```python
from build123d import *

# Parameters (mm, degrees)
CYLINDER003012_R     = 0.93
CYLINDER003012_DEPTH = 20
CYLINDER003013_R     = 2.4
CYLINDER003013_DEPTH = 4.5
CYLINDER003014_R     = 3.45
CYLINDER003014_DEPTH = 4.5


with BuildPart() as cylinder013:
    # Cylinder003012 → Cylinder003012 (new body)
    with BuildSketch(Plane(origin=(11, 10, -8), x_dir=(1, 0, 0), z_dir=(0, 0, 1))):
        Circle(CYLINDER003012_R)
    extrude(amount=CYLINDER003012_DEPTH)


with BuildPart() as cylinder014:
    # Cylinder003013 → Cylinder003013 (new body)
    with BuildSketch(Plane(origin=(11, 10, -0.5), x_dir=(1, 0, 0), z_dir=(0, 0, 1))):
        Circle(CYLINDER003013_R)
    extrude(amount=CYLINDER003013_DEPTH)


with BuildPart() as propeller_hub:
    # Cylinder003014 → Cylinder003014 (new body)
    with BuildSketch(Plane(origin=(11, 10, -4.5), x_dir=(1, 0, 0), z_dir=(0, 0, 1))):
        Circle(CYLINDER003014_R)
    extrude(amount=CYLINDER003014_DEPTH)

    # Fusion001: union Cylinder014
    add(cylinder014.part)

    # Cut002002002018: cut Cylinder013
    add(cylinder013.part, mode=Mode.SUBTRACT)


solid = propeller_hub.part
```
Verification items for the finished model (mm, model axes). A direction names the side the tool comes from. Coordinates: 2 decimals unless noted, no trailing zeros. Order: outer loops, then holes, each group sorted by start corner. A loop starts at its lowest first (then second) coordinate and runs counter-clockwise, first axis right, second up. Notation, with made-up numbers: (73.25, 34.5) -> (85.25, 34.5) arc R5 ccw to (85.25, 43.5) -> close; hole circle Ø7 at (-4.75, 63.25). An arc over 180 degrees is marked (long way). Put each result on its own line as item: value. Start each with the question number.
1) Tool access check on faces 4 (the flat face through (12, 9, -4.5)), 5 (the cylindrical face through (10.69, 12.38, 1.97)). Record the directions out of +Z, -Z, +X, -X, +Y, -Y that give a thin tool (end or side, any length) a straight path to the whole face; none if there is none.
2) Release check for a two-part mould opening along X. For faces 1 (the cylindrical face through (10.252, 6.632, -2.282)), 2 (the cylindrical face through (11.5, 10.784, -0.309)), 3 (the flat face through (12, 9.5, 4)) record: pulls with the +X half, pulls with the -X half, needs draft (parallel to the pull), parting line crosses it, or undercut.
3) Cross-section at D-D (y = 8). Enter the section's corners in (x, z).
4) Material ranges on L1, parallel to Y at x = 11, z = -1; L2, parallel to Z at x = 12.75, y = 12.5; L3, parallel to X at y = 10, z = 0.5, recorded low to high.
5) Cross-section at C-C (z = -2.5). Enter the section's corners in (x, y), plus the area to 3 significant figures.
6) Cross-section at B-B (y = 10). Enter the section's corners in (x, z).
7) Cross-section at A-A (x = 11). Enter the section's corners in (y, z).
Geometry check:
1. face 4: -Z, +X, -X, +Y, -Y
1. face 5: +Z
2. face 1: parting line crosses it
2. face 2: undercut
2. face 3: needs draft
3. outline: (8.19, -4.5) -> (13.81, -4.5) -> (13.81, 0) -> (12.33, 0) -> (12.33, 4) -> (9.67, 4) -> (9.67, 0) -> (8.19, 0) -> close
4. L1: y = 6.55 to 9.07, 10.93 to 13.45
4. L2: z = -4.5 to 0
4. L3: x = 8.6 to 10.07, 11.93 to 13.4
5. outline: circle Ø6.9 at (11, 10); hole circle Ø1.86 at (11, 10)
5. area: 34.7 mm^2
6. outline: (7.55, -4.5) -> (10.07, -4.5) -> (10.07, 4) -> (8.6, 4) -> (8.6, 0) -> (7.55, 0) -> close; (11.93, -4.5) -> (14.45, -4.5) -> (14.45, 0) -> (13.4, 0) -> (13.4, 4) -> (11.93, 4) -> close
7. outline: (6.55, -4.5) -> (9.07, -4.5) -> (9.07, 4) -> (7.6, 4) -> (7.6, 0) -> (6.55, 0) -> close; (10.93, -4.5) -> (13.45, -4.5) -> (13.45, 0) -> (12.4, 0) -> (12.4, 4) -> (10.93, 4) -> close
